```python
from build123d import *

# Parameters (mm, degrees)
F0_W     = 100
F0_H     = 50
F2_T     = -2.5
F3_R     = 432.257955
F4_DEPTH = 2.501


with BuildPart() as f1:
    # F0 (on Right) → F1 (revolve)
    with BuildSketch(Plane.YZ):
        Polygon((-220, 0), (0, 0), (0, 340), (-445, 340), (-445, 0), (-320, 0), (-320, 50), (-220, 50), align=None)
        with Locations((-270, 25)):
            Rectangle(F0_W, F0_H)
    revolve(axis=Axis((0, 0, 170), (0, 0, 1)))

    # F2
    f2_openings = [f1.faces().sort_by_distance(p)[0] for p in [
        (0, 0, 340),
    ]]
    offset(amount=F2_T, openings=f2_openings)

    # F3 (on face) → F4 (cut, through all)
    with BuildSketch(Plane.XY.offset(2.5)):
        Circle(F3_R)
    extrude(amount=-F4_DEPTH, mode=Mode.SUBTRACT)


solid = f1.part
```
Build history of the part. All positions in model axes, mm. Round coordinates to 2 decimals unless told otherwise and drop trailing zeros. Order: outer loops, then holes, each group sorted by start corner. A loop starts at its lowest first (then second) coordinate and runs counter-clockwise, first axis right, second up. Notation, with made-up numbers: (35, 50) - (47, 50) arc R12 cw to (47, 59) - close; hole circle Ø1 at (89, 66.25). An arc over 180 degrees is marked (long way). Use a Markdown table: item, result.
1) Wall check: L1, parallel to X at y = 0, z = 217.5; L2, parallel to Y at x = 165, z = 50; L3, parallel to X at y = 107, z = 259.5. Give the ranges that are in metal, low to high.
Recorded:
| item | result |
|---|---|
| L1 | x = -445 to -442.5, 442.5 to 445 |
| L2 | y = -413.28 to -410.59, 410.59 to 413.28 |
| L3 | x = -431.94 to -429.37, 429.37 to 431.94 |
2) Saw through at C-C on z = 212. Write the cut outline in (x, y).
Recorded:
| item | result |
|---|---|
| outline | circle Ø890 at (0, 0); hole circle Ø885 at (0, 0) |
3) Saw through at A-A on y = 0. Write the cut outline in (x, z).
Recorded:
| item | result |
|---|---|
| outline | (-445, 0) - (-432.26, 0) - (-432.26, 2.5) - (-442.5, 2.5) - (-442.5, 340) - (-445, 340) - close; (432.26, 0) - (445, 0) - (445, 340) - (442.5, 340) - (442.5, 2.5) - (432.26, 2.5) - close |
4) Pull direction Y, two halves, no side cores. Call faces 1 (the face through (232.38, 364.48, 1.27)), 2 (the face through (132.915, -422.066, 168.888)), 3 (the face through (441.213, 57.93, 167.62)), 4 (the face through (365, 233, 0)): pulls with the +Y half, pulls with the -Y half, needs draft (parallel to the pull), parting line crosses it, or undercut.
Recorded:
| item | result |
|---|---|
| face 1 | undercut |
| face 2 | undercut |
| face 3 | parting line crosses it |
| face 4 | needs draft |
5) Flat gauge pins, fed straight in: pin 1 Ø2 at (y, z) = (-209, 159) entering from +X; pin 2 Ø8 at (x, z) = (116, 133) entering from -Y; pin 3 Ø8 at (x, z) = (-241.5, 123.5) entering from -Y. Where does each tip first touch, or does it go through?
Recorded:
| item | result |
|---|---|
| pin 1 | stops at x = 393.4 |
| pin 2 | stops at y = -430.68 |
| pin 3 | stops at y = -376.32 |
